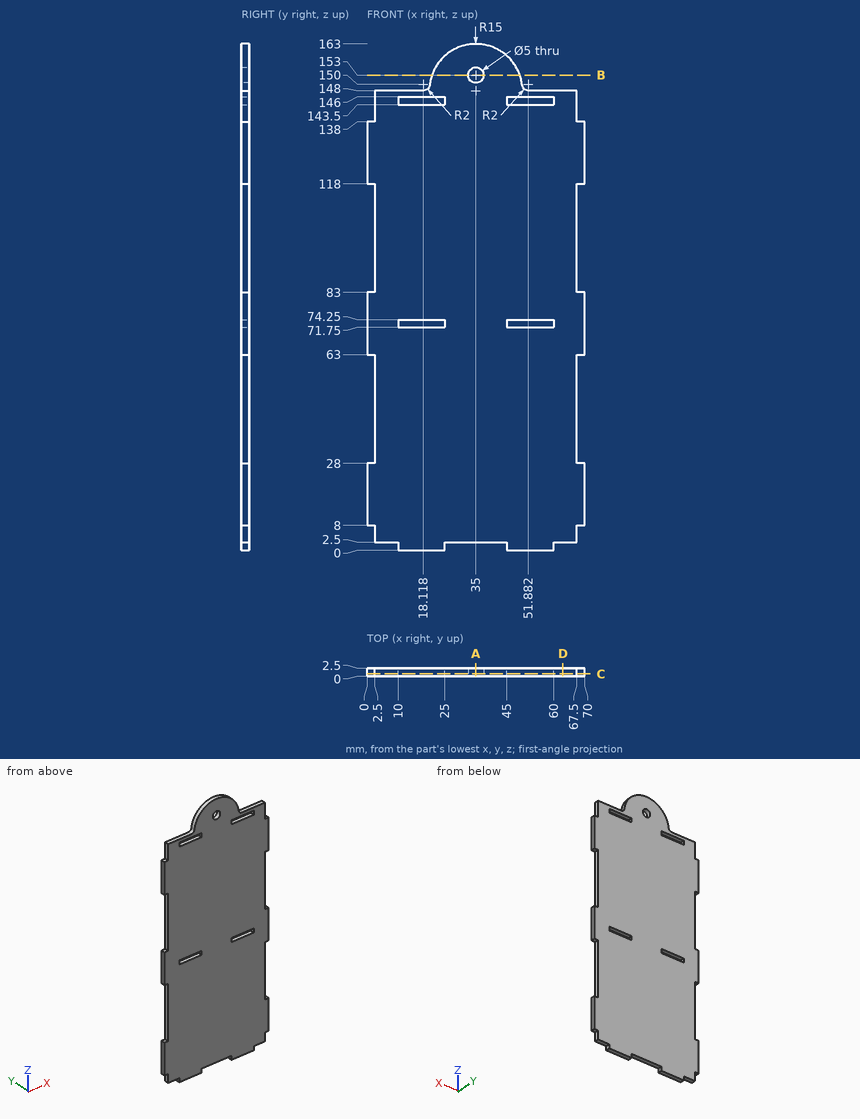
Geometry: see drawing. Coordinates: mm, zero at the bounding-box minimum. Coordinates: 2 decimals unless noted, no trailing zeros. Loops run counter-clockwise (first coordinate to the right, second up) from the corner with the lowest first, then second, coordinate; pieces in that order, holes last. Notation, with made-up numbers: (85.25, -13) -> (141.25, -13) arc R13 cw to (141.25, 10) -> close; hole circle Ø4 at (14.5, -29.75). An arc over 180 degrees is marked (long way). Write item = value, one per line. Start each with the question number.
Item 1: First-contact query: P1, Ø1, axis at x = 55.5, y = 1.5, coming from the -Z side; P2, Ø1.2, axis at y = 0.5, z = 5.5, coming from the -X side; P3, Ø1.2, axis at y = 0.5, z = 1.5, coming from the +X side. Flat tips, straight axial feed; report the tip coordinate or a pass-through.
Item 2: Cut plane B-B, the plane z = 153. Return loops of the section in (x, y).
Item 3: Cut plane D-D, the plane x = 63. Return loops of the section in (y, z), plus the area to 3 significant figures.
Item 4: Material intervals for line 1 (Z direction, x = 12, y = 0.7); line 2 (X direction, y = 1.8, z = 153); line 3 (X direction, y = 1, z = 88), sorted ascending.
Item 5: Cut plane C-C, the plane y = 0.65. Count the separate pieces of the cut face and the enclosed holes in it, plus the area to 3 significant figures.
Item 6: Cut plane A-A, the plane x = 35. Return loops of the section in (y, z), plus the area to 3 significant figures.
Ans:
q1.P1 = 0
q1.P2 = 2.5
q1.P3 = 60
q2.outline = (20.86, 0) -> (32.5, 0) -> (32.5, 2.5) -> (20.86, 2.5) -> close; (37.5, 0) -> (49.14, 0) -> (49.14, 2.5) -> (37.5, 2.5) -> close
q3.outline = (0, 2.5) -> (2.5, 2.5) -> (2.5, 148) -> (0, 148) -> close
q3.area = 364 mm²
q4.line_1 = 0 to 71.75, 74.25 to 143.5, 146 to 148
q4.line_2 = 20.86 to 32.5, 37.5 to 49.14
q4.line_3 = 2.5 to 67.5
q5.separate_pieces = 1
q5.enclosed_holes = 5
q5.area = 10,000 mm²
q6.outline = (0, 2.5) -> (2.5, 2.5) -> (2.5, 150.5) -> (0, 150.5) -> close; (0, 155.5) -> (2.5, 155.5) -> (2.5, 163) -> (0, 163) -> close
q6.area = 389 mm²
